Solid Edge part; units mm, degrees
sketch "Sketch1" plane through (0, 0, 0) normal (0, 0, 1) x (1, 0, 0)
  line L0 (-6, 10.5) -> (-30, 10.5)
  line L1 (-30, 10.5) -> (-30, 14)
  line L2 (-30, 14) -> (0, 14)
  line L3 (0, 14) -> (0, 6)
  line L4 (0, 6) -> (-6, 6)
  line L5 (-6, 6) -> (-6, 10.5)
revolve "RevolvedProtrusion1" add sketch "Sketch1" angle 360 about axis through (-24.1113, 0, 0) along (1, 0, 0)
sketch "Sketch2" plane through (0, 0, 0) normal (0, -1, 0) x (1, 0, 0)
  line L0 (-30, 12.1801) -> (-25, 14)
revolve "RevolvedCutout1" cut sketch "Sketch2" angle 360 about axis through (-24.1113, 0, 0) along (1, 0, 0) material side at (-27.5171, 0, 13.137)
Verification items for the finished model (mm, model axes). Coordinates: 2 decimals unless noted, no trailing zeros. Order: outer loops, then holes, each group sorted by start corner. A loop starts at its lowest first (then second) coordinate and runs counter-clockwise, first axis right, second up.
Item 1: Section check C-C, the plane x = -23.25. Enter the section's corners in (y, z), then the cut area to 3 significant figures.
Filled in:
outline: circle Ø28 at (0, 0); hole circle Ø21 at (0, 0)
area: 269 mm2
Item 2: Depth check by flat-ended pin: pin 1 (2 mm diameter, centred on x = -6.5, z = 10, fed in from -Y); pin 2 (2 mm diameter, centred on x = -25, z = -3, fed in from -Y). Enter the tip coordinate at first touch or a pass-through.
Filled in:
pin 1: stops at y = -10.72
pin 2: stops at y = -13.86
Item 3: Release check for a two-part mould opening along Z. For faces 1 (the face through (-18.2, 10, -3.2)), 2 (the face through (-6, 5, -5)), 3 (the face through (-30, 4, 10)), 4 (the face through (-12.325, 12.932, -5.362)) record: +Z half, -Z half, draft (parallel to the pull), parting line (faces both ways), or undercut.
Filled in:
face 1: undercut
face 2: undercut
face 3: draft
face 4: parting line
Item 4: Material ranges on L1, parallel to Z at x = -23.5, y = 0; L2, parallel to Z at x = -4.45, y = 0; L3, parallel to X at y = 9.25, z = -0.25, recorded low to high.
Filled in:
L1: z = -14 to -10.5, 10.5 to 14
L2: z = -14 to -6, 6 to 14
L3: x = -6 to 0
Item 5: Section check A-A, the plane z = 0. Enter the section's corners in (x, y), then the cut area to 3 significant figures.
Filled in:
outline: (-30, -12.18) - (-25, -14) - (0, -14) - (0, -6) - (-6, -6) - (-6, -10.5) - (-30, -10.5) - close; (-30, 10.5) - (-6, 10.5) - (-6, 6) - (0, 6) - (0, 14) - (-25, 14) - (-30, 12.18) - close
area: 255 mm2
